```python
from build123d import *

# Parameters (mm, degrees)
SKETCH1_R                                          = 51.054
SKETCH1_R_2                                        = 28.702
BOSS_EXTRUDE1_DEPTH                                = 7.62
CSK_FOR_10_FLAT_HEAD_MACHINE_SCREW_100_D           = 4.9784
CSK_FOR_10_FLAT_HEAD_MACHINE_SCREW_100_CSINK_D     = 9.779
CSK_FOR_10_FLAT_HEAD_MACHINE_SCREW_100_CSINK_ANGLE = 100
CIRPATTERN1_COUNT                                  = 3
SKETCH6_R                                          = 51.054
SKETCH6_R_2                                        = 49.53
CUT_EXTRUDE1_DEPTH                                 = 2.54


with BuildPart() as part:
    # Sketch1 → Boss-Extrude1 (new body)
    with BuildSketch(Plane(origin=(0, 0, 0), x_dir=(1, 0, 0), z_dir=(0, 1, 0))):
        with Locations(Location((0, 0, 0), (0, 0, 90))):
            Circle(SKETCH1_R)
        with Locations(Location((0, 0, 0), (0, 0, 90))):
            Circle(SKETCH1_R_2, mode=Mode.SUBTRACT)
    extrude(amount=BOSS_EXTRUDE1_DEPTH)

    # CSK for #10 Flat Head Machine Screw (100)1 (through all)
    with Locations(Plane(origin=(0, 7.62, 0), x_dir=(1, 0, 0), z_dir=(0, 1, 0))):
        with Locations((44.45, 0)):
            csk_for_10_flat_head_machine_screw_100 = CounterSinkHole(CSK_FOR_10_FLAT_HEAD_MACHINE_SCREW_100_D / 2, CSK_FOR_10_FLAT_HEAD_MACHINE_SCREW_100_CSINK_D / 2, counter_sink_angle=CSK_FOR_10_FLAT_HEAD_MACHINE_SCREW_100_CSINK_ANGLE)

    # CirPattern1: CSK for #10 Flat Head Machine Screw (100)1 ×3 about axis
    cirpattern1_axis = Axis((0, 0, 0), (0, 1, 0))
    for i in range(1, CIRPATTERN1_COUNT):
        add(csk_for_10_flat_head_machine_screw_100.rotate(cirpattern1_axis, i * 360 / CIRPATTERN1_COUNT), mode=Mode.SUBTRACT)

    # Sketch6 → Cut-Extrude1 (cut)
    with BuildSketch(Plane.XZ):
        with Locations(Location((0, 0, 0), (0, 0, 270))):
            Circle(SKETCH6_R)
        with Locations(Location((0, 0, 0), (0, 0, 270))):
            Circle(SKETCH6_R_2, mode=Mode.SUBTRACT)
    extrude(amount=-CUT_EXTRUDE1_DEPTH, mode=Mode.SUBTRACT)


solid = part.part
```
Part model, mm, in its own coordinate system. A direction names the side the tool comes from. Round coordinates to 2 decimals unless told otherwise and drop trailing zeros. Order: outer loops, then holes, each group sorted by start corner. A loop starts at its lowest first (then second) coordinate and runs counter-clockwise, first axis right, second up. Notation, with made-up numbers: M -21.75,-35.5 L -7.75,-35.5 A17 cw -7.75,-26.5 Z; hole C -9,84 d7. An arc over 180 degrees is marked long. Put each result on its own line as item: value. Start each with the question number.
1. Drop flat-ended pins along their axis: pin 1 (1.5 mm diameter, centred on x = 29.5, z = 24.5, fed in from -Y); pin 2 (2 mm diameter, centred on x = 4.5, y = 6, fed in from -Z); pin 3 (1.5 mm diameter, centred on x = -22.5, y = 4.5, fed in from -Z); pin 4 (5.5 mm diameter, centred on x = -22.23, z = 38.49, fed in from +Y). Give the stop position or say it passes through.
2. Two-plate mould, pull along X, no slides. Class faces 3 (the face through (-20.25, 2.76, 40.01)), 4 (the face through (27, 2.54, 42)), 5 (the face through (19.554, 5.044, -47.161)), 6 (the face through (10.993, 3.757, -26.513)): +X half, -X half, draft (parallel to the pull), parting line (faces both ways), or undercut.
3. Slice it at A-A on z = 0. List the corners of the cut face in (x, y), then the cut area to 3 significant figures.
4. Slice it at B-B on x = 0. List the corners of the cut face in (y, z).
5. Slice it at D-D on z = -30.5. List the corners of the cut face in (x, y).
6. Slice it at C-C on z = -19. List the corners of the cut face in (x, y).
7. Tool access for faces 1 (the face through (14.88, 1.25, -47.24)), 2 (the face through (-23.626, 5.704, -40.692)): list every direction of +Z, -Z, +X, -X, +Y, -Y with a clear straight run to the whole face (end or side of a thin tool).
8. Drill centre lines: probe 1 along Z at (x, y) = (1, 2); probe 2 along X at (y, z) = (5.25, -17); probe 3 along Z at (x, y) = (14.5, 6). Where is each one in solid material? Low to high. Write a range as [from, to].
Findings:
1. pin 1: y = 0
1. pin 2: z = -50.93
1. pin 3: z = -46.19
1. pin 4: y = 5.83
2. face 3: undercut
2. face 4: draft
2. face 5: parting line
2. face 6: undercut
3. outline: M -51.05,2.54 L -49.53,2.54 L -49.53,0 L -28.7,0 L -28.7,7.62 L -51.05,7.62 Z; M 28.7,0 L 41.96,0 L 41.96,5.61 L 39.56,7.62 L 28.7,7.62 Z; M 46.94,0 L 49.53,0 L 49.53,2.54 L 51.05,2.54 L 51.05,7.62 L 49.34,7.62 L 46.94,5.61 Z
3. area: 290 mm2
4. outline: M 0,-49.53 L 2.54,-49.53 L 2.54,-51.05 L 7.62,-51.05 L 7.62,-28.7 L 0,-28.7 Z; M 0,28.7 L 7.62,28.7 L 7.62,51.05 L 2.54,51.05 L 2.54,49.53 L 0,49.53 Z
5. outline: M -40.94,2.54 L -39.03,2.54 L -39.03,0 L 39.03,0 L 39.03,2.54 L 40.94,2.54 L 40.94,7.62 L -40.94,7.62 Z
6. outline: M -47.39,2.54 L -45.74,2.54 L -45.74,0 L -21.51,0 L -21.51,7.62 L -47.39,7.62 Z; M 21.51,0 L 45.74,0 L 45.74,2.54 L 47.39,2.54 L 47.39,7.62 L 21.51,7.62 Z
7. face 1: -Y
7. face 2: +Y
8. probe 1: [-49.52, -28.68], [28.68, 49.52]
8. probe 2: [-48.14, -23.13], [23.13, 48.14]
8. probe 3: [-48.95, -24.77], [24.77, 48.95]
